```python
from build123d import *

# Parameters (mm, degrees)
SKETCH_1_W          = 130
SKETCH_1_H          = 30
EXTRUDE_1_DEPTH     = 180
SKETCH_2_R          = 38.5
SKETCH_2_R_2        = 33.5
EXTRUDE_1_2_DEPTH   = 70
SKETCH_3_R          = 45
CUT_EXTRUDE_1_DEPTH = 25
SKETCH_5_R          = 33.5
EXTRUDE_2_DEPTH     = 20
SKETCH_4_R          = 20
CUT_EXTRUDE_2_DEPTH = 40
SKETCH_7_W          = 10
SKETCH_7_H          = 10
CUT_EXTRUDE_3_DEPTH = 130
SKETCH_8_W          = 18.558998623
SKETCH_8_H          = 76.555219483
CUT_EXTRUDE_4_DEPTH = 40
FILLET_START        = 5
FILLET_1_2_DEPTH    = 10


with BuildPart() as part:
    # 草图1 → Extrude 1 (new body)
    with BuildSketch(Plane.XY):
        with Locations((0, 15)):
            Rectangle(SKETCH_1_W, SKETCH_1_H)
    extrude(amount=-EXTRUDE_1_DEPTH)

    # 草图2 → Extrude 1 2 (add)
    with BuildSketch(Plane(origin=(0, 30, 0), x_dir=(1, 0, 0), z_dir=(0, 1, 0))):
        with Locations((0, 140)):
            Circle(SKETCH_2_R)
        with Locations((0, 140)):
            Circle(SKETCH_2_R_2, mode=Mode.SUBTRACT)
    extrude(amount=EXTRUDE_1_2_DEPTH)

    # 草图3 → 切除-拉伸1 (cut)
    with BuildSketch(Plane(origin=(0, 30, 0), x_dir=(1, 0, 0), z_dir=(0, 1, 0))):
        with Locations(Location((0, 49.571769675, 0), (0, 0, 270))):
            Circle(SKETCH_3_R)
    extrude(amount=-CUT_EXTRUDE_1_DEPTH, mode=Mode.SUBTRACT)

    # 草图5 → 凸台-拉伸2 (add)
    with BuildSketch(Plane(origin=(0, 30, 0), x_dir=(1, 0, 0), z_dir=(0, 1, 0))):
        with Locations(Location((0, 140, 0), (0, 0, 270))):
            Circle(SKETCH_5_R)
    extrude(amount=EXTRUDE_2_DEPTH)

    # 草图4 → 切除-拉伸2 (cut)
    with BuildSketch(Plane(origin=(0, 50, 0), x_dir=(1, 0, 0), z_dir=(0, 1, 0))):
        with Locations(Location((0, 140, 0), (0, 0, 270))):
            Circle(SKETCH_4_R)
    extrude(amount=-CUT_EXTRUDE_2_DEPTH, mode=Mode.SUBTRACT)

    # 草图7 → 切除-拉伸3 (cut)
    with BuildSketch(Plane.XY.offset(-20)):
        with Locations((0, 10)):
            Rectangle(SKETCH_7_W, SKETCH_7_H)
    extrude(amount=-CUT_EXTRUDE_3_DEPTH, mode=Mode.SUBTRACT)

    # 草图8 → 切除-拉伸4 (cut)
    with BuildSketch(Plane(origin=(65, 0, 0), x_dir=(0, 0, -1), z_dir=(1, 0, 0))):
        with Locations((142.072443273, 68.277609742)):
            Rectangle(SKETCH_8_W, SKETCH_8_H)
    extrude(amount=-CUT_EXTRUDE_4_DEPTH, mode=Mode.SUBTRACT)

    # 圆角1: read off the stored shape, not the designer's step
    # 圆角1 outline → 圆角1 (revolve)
    with BuildSketch(Plane.XY.offset(-49.571769675)):
        with BuildLine():
            ThreePointArc((45, 15), (42.071067812, 7.928932188), (35, 5))
            Line((35, 5), (45, 5))
            Line((45, 5), (45, 15))
        make_face()
    revolve(axis=Axis((0, 0, -49.571769675), (0, 1, 0)))

    # Fillet 1 2 outline → Fillet 1 2 (cut)
    with BuildSketch(Plane(origin=(0, 0, 0), x_dir=(1, 0, 0), z_dir=(0, 1, 0)).offset(FILLET_START)):
        with BuildLine():
            Line((-5, 150), (-5, 84.212785827))
            ThreePointArc((-5, 84.212785827), (0, 14.571769675), (5, 84.212785827))
            Line((5, 84.212785827), (5, 150))
            Line((5, 150), (-5, 150))
        make_face()
    extrude(amount=FILLET_1_2_DEPTH, mode=Mode.SUBTRACT)


solid = part.part
```
Input: part model. Units: mm. Frame: model coordinates. A direction names the side the tool comes from. Coordinates: 2 decimals unless noted, no trailing zeros. Loops run counter-clockwise (first coordinate to the right, second up) from the corner with the lowest first, then second, coordinate; pieces in that order, holes last. Notation, with made-up numbers: M 43.5,65.25 L 78.5,65.25 A31 ccw 78.5,94.25 Z; hole C 41.25,19.5 d7. An arc over 180 degrees is marked long. Answer in a Markdown table with one row per item.
1. Section D-D, the plane z = -114. Output: boundary loops of the cut face in (x, y).
Response:
| item | result |
|---|---|
| outline | M -65,0 L 65,0 L 65,30 L 28.39,30 L 28.39,100 L 21.12,100 L 21.12,50 L -21.12,50 L -21.12,100 L -28.39,100 L -28.39,30 L -65,30 Z; hole M -5,5 L 5,5 L 5,15 L -5,15 Z |
2. Section B-B, the plane z = -140. Output: boundary loops of the cut face in (x, y), then the cut area to 3 significant figures.
Response:
| item | result |
|---|---|
| outline | M -65,0 L 65,0 L 65,30 L 25,30 L 25,50 L 20,50 L 20,10 L 5,10 L 5,5 L -5,5 L -5,10 L -20,10 L -20,50 L -33.5,50 L -33.5,100 L -38.5,100 L -38.5,30 L -65,30 Z |
| area | 3,770 mm2 |
3. Reachability of faces 4 (the flat face through (-15, 50, -126)), 5 (the flat face through (25, 40, -142)), 6 (the flat face through (-1, 15, -180)), 7 (the flat face through (5, 9, -117)) from +Z, -Z, +X, -X, +Y, -Y: full face, straight path, thin tool, end or side. Return the list, or none.
Response:
| item | result |
|---|---|
| face 4 | +Y |
| face 5 | +X, +Y |
| face 6 | -Z, +X, -X, +Y, -Y |
| face 7 | none |
4. First-contact query: pin 1 (1 mm diameter, centred on x = 15, y = 77, fed in from -Z); pin 2 (9.5 mm diameter, centred on y = 40, z = -138, fed in from +X); pin 3 (14 mm diameter, centred on x = 34, y = 62, fed in from -Z). Flat tips, straight axial feed; report the tip coordinate or a pass-through.
Response:
| item | result |
|---|---|
| pin 1 | stops at z = -175.67 |
| pin 2 | stops at x = 25 |
| pin 3 | stops at z = -167.45 |
5. Section A-A, the plane x = 0. Output: boundary loops of the cut face in (y, z).
Response:
| item | result |
|---|---|
| outline | M 0,-180 L 30,-180 L 30,-178.5 L 100,-178.5 L 100,-173.5 L 50,-173.5 L 50,-160 L 10,-160 L 10,-150 L 5,-150 L 5,-14.57 A10 cw 15,-4.57 L 30,-4.57 L 30,0 L 0,0 Z; M 15,-120 L 50,-120 L 50,-106.5 L 100,-106.5 L 100,-101.5 L 30,-101.5 L 30,-94.57 L 15,-94.57 Z |
6. Material intervals for line 1 (Z direction, x = 0, y = 21.25); line 2 (Z direction, x = 0, y = 72.5); line 3 (X direction, y = 34, z = -140), sorted ascending.
Response:
| item | result |
|---|---|
| line 1 | z = -180 to -160, -120 to -94.57, -4.57 to 0 |
| line 2 | z = -178.5 to -173.5, -106.5 to -101.5 |
| line 3 | x = -38.5 to -20, 20 to 25 |
7. Section C-C, the plane y = 41. Output: boundary loops of the cut face in (x, z).
Response:
| item | result |
|---|---|
| outline | M 25,-151.35 L 25,-132.79 L 37.82,-132.79 A38.5 ccw long 36.79,-151.35 Z; hole C 0,-140 d40 |
8. Draft query along X for faces 1 (the cylindrical face through (-38.496, 64.51, -139.425)), 2 (the flat face through (-5, 9, -118)), 3 (the flat face through (-1, 0, -89)). Return one class per face: pulls with the +X half, pulls with the -X half, needs draft (parallel to the pull), parting line crosses it, or undercut.
Response:
| item | result |
|---|---|
| face 1 | parting line crosses it |
| face 2 | undercut |
| face 3 | needs draft |
